Verification items for the finished model (mm, model axes). A direction names the side the tool comes from. Give positions to 0.01 mm unless a question says otherwise; leave off trailing zeros. Order: outer loops, then holes, each group sorted by start corner. A loop starts at its lowest first (then second) coordinate and runs counter-clockwise, first axis right, second up. Notation, with made-up numbers: M 30,74.5 L 84,74.5 A14 ccw 84,101.5 Z; hole C 7,-36.75 d6. An arc over 180 degrees is marked long. Answer as a JSON object with one key per item and string values.
```python
from build123d import *

# Parameters (mm, degrees)
F0_W        = 87.5
F0_H        = 19.5
F0_W_2      = 84.5
F0_H_2      = 16.5
F1_DEPTH    = 30
F2_DEPTH    = 3
F3_SIZE     = 1
F5_DEPTH    = 25
F6_DEPTH    = 25
F7_T1_DEPTH = 40.3581649162


# Not quite as in the source:
# - a fillet or chamfer that OpenCascade refuses, or shapes differently, is made with other operations: its cross-section is extruded or revolved along the edge and cut away or added


with BuildPart() as f1:
    # F0 (on Top) → F1 (new body)
    with BuildSketch(Plane.XY):
        Rectangle(F0_W, F0_H)
        Rectangle(F0_W_2, F0_H_2, mode=Mode.SUBTRACT)
    extrude(amount=F1_DEPTH)

    # F0 (on Top) → F2 (join)
    with BuildSketch(Plane.XY):
        Rectangle(F0_W_2, F0_H_2)
    extrude(amount=F2_DEPTH)

    # F3
    f3_edges = [f1.edges().sort_by_distance(p)[0] for p in [
        (-43.75, -9.75, 15),
        (43.75, -9.75, 15),
    ]]
    chamfer(f3_edges, length=F3_SIZE)

    # F4 (on face) → F5 (join)
    with BuildSketch(Plane.XY.offset(30)):
        Polygon((-43.75, 9.75), (-43.75, 0), (-42.25, 0), (-42.25, 8.25), (42.25, 8.25), (42.25, 0), (43.75, 0), (43.75, 9.75), align=None)
    extrude(amount=F5_DEPTH)

    # F4 (on face) → F6 (cut)
    with BuildSketch(Plane.XY.offset(30)):
        Polygon((50.0001870096, 0), (-45.6664785743, 0), (-48.1942594051, -2.8349049389), (-42.25, -20.2376823872), (42.25, -19.071014598), align=None)
    extrude(amount=F6_DEPTH, mode=Mode.SUBTRACT)

    # F7: chamfer of 5 x 5.958767963 on 2 edges, made by hand

    # F7_s2 → F7_t1 (cut)
    with BuildSketch(Plane.XY.offset(30)):
        Polygon((-43.75, 5.958767963), (-38.75, 0), (-43.75, 0), align=None)
        Polygon((43.75, 5), (37.791232037, 0), (43.75, 0), align=None)
    extrude(amount=F7_T1_DEPTH, mode=Mode.SUBTRACT)


solid = f1.part
```
Q1. Section check C-C on z = 18. Record the cut outline in (x, y).
Resolved:
{"outline": "M -43.75,-8.75 L -42.75,-9.75 L 42.75,-9.75 L 43.75,-8.75 L 43.75,9.75 L -43.75,9.75 Z; hole M -42.25,-8.25 L 42.25,-8.25 L 42.25,8.25 L -42.25,8.25 Z"}
Q2. Section check A-A on x = 19.5. Record the cut outline in (y, z).
Resolved:
{"outline": "M -9.75,0 L 9.75,0 L 9.75,55 L 8.25,55 L 8.25,3 L -8.25,3 L -8.25,30 L -9.75,30 Z"}
Q3. Tool access check on faces 4 (the face through (-1, -8.25, 16)), 5 (the face through (-1, 0, 0)). Record the directions out of +Z, -Z, +X, -X, +Y, -Y that give a thin tool (end or side, any length) a straight path to the whole face; none if there is none.
Resolved:
{"face 4": "+Z", "face 5": "-Z, +X, -X, +Y, -Y"}
Q4. Gauge pin test, flat ends, axial feed: pin 1 Ø10 at (x, y) = (34, -6) entering from +Z; pin 2 Ø4.5 at (x, y) = (-3.5, 1.5) entering from +Z. Record the tip position at first contact, or that the pin passes through.
Resolved:
{"pin 1": "stops at z = 30", "pin 2": "stops at z = 3"}
Q5. Release check for a two-part mould opening along X. For faces 1 (the face through (-1, -9.75, 15)), 2 (the face through (-1, 8.25, 29)), 3 (the face through (-43.01, 5.077, 42.325)) record: +X half, -X half, draft (parallel to the pull), parting line (faces both ways), or undercut.
Resolved:
{"face 1": "draft", "face 2": "undercut", "face 3": "-X half"}
Q6. Section check B-B on z = 35.5. Record the cut outline in (x, y), then the cut area to 3 significant figures.
Resolved:
{"outline": "M -43.75,5.96 L -42.25,4.17 L -42.25,8.25 L 42.25,8.25 L 42.25,3.74 L 43.75,5 L 43.75,9.75 L -43.75,9.75 Z", "area": "142 mm²"}
Q7. Material ranges on L1, parallel to X at y = -4.25, z = 23; L2, parallel to Y at x = -37, z = 15; L3, parallel to Y at x = -24, z = 38.5, recorded low to high.
Resolved:
{"L1": "x = -43.75 to -42.25, 42.25 to 43.75", "L2": "y = -9.75 to -8.25, 8.25 to 9.75", "L3": "y = 8.25 to 9.75"}
